Check sheet for the modelled part. Datum: model origin and axes. Units: mm. A direction names the side the tool comes from. Round coordinates to 2 decimals unless told otherwise and drop trailing zeros. Loops run counter-clockwise (first coordinate to the right, second up) from the corner with the lowest first, then second, coordinate; pieces in that order, holes last. Notation, with made-up numbers: (73, 5) - (87, 5) arc R16 cw to (87, 14) - close; hole circle Ø5 at (81.5, 48). An arc over 180 degrees is marked (long way). Put each result on its own line as item: value. Start each with the question number.
Item 1: Draft check along X on faces 4 (the conical face through (-34.97, -0.09, 75.19)), 5 (the conical face through (-37.42, -0.09, 77.21)), 6 (the flat face through (6.123, 34.723, 75.862)). Enter one of: pulls with the +X half, pulls with the -X half, needs draft (parallel to the pull), parting line crosses it, or undercut.
Item 2: Section check C-C, the plane x = -18.5. Record the cut outline in (y, z), and give its area (3 significant figures).
Item 3: Gauge pin test, flat ends, axial feed: pin 1 Ø23 at (x, y) = (-13, -16) entering from -Z; pin 2 Ø5 at (x, z) = (4.5, 47.5) entering from -Y; pin 3 Ø4 at (x, z) = (1.5, 152) entering from +Y (3 decimals); pin 4 Ø1.5 at (x, z) = (-31.5, 93.5) entering from +Y. Record the tip position at first contact, or that the pin passes through.
Item 4: Material ranges on line 1 along Y through (x, z) = (0, 154) (3 decimals); line 2 along Y through (x, z) = (0, -1.75) (3 decimals); line 3 along X through (y, z) = (0, 0), recorded low to high.
Item 5: Section check B-B, the plane y = 0. Record the cut outline in (x, z).
Item 6: Section check D-D, the plane y = -27. Record the cut outline in (x, z), and give its area (3 significant figures).
Item 7: Tool access check on faces 1 (the flat face through (-35.99, 6.346, 75.862)), 2 (the flat face through (0, 38.735, 0)), 3 (the conical face through (34.97, 0.09, 75.19)). Record the directions out of +Z, -Z, +X, -X, +Y, -Y that give a thin tool (end or side, any length) a straight path to the whole face; none if there is none.
Item 8: Section check A-A, the plane z = 110. Record the cut outline in (x, y).
from build123d import *

# Parameters (mm, degrees)
SKETCH1_R                      = 40.64
SKETCH1_R_2                    = 38.1
BOSS_EXTRUDE1_DEPTH            = 3.81
CUT_EXTRUDE1_REACH             = 5.81
SKETCH2_W                      = 7.62
SKETCH2_H                      = 3.81
CUT_EXTRUDE1_DIRECTION_2_REACH = 5.81
SKETCH3_R                      = 34.29
SKETCH3_R_2                    = 31.75
BOSS_EXTRUDE2_DEPTH            = 3.81
REVOLVE1_ANGLE                 = 10
REVOLVE1_OTHER_WAY_ANGLE       = 10
CUT_EXTRUDE2_REACH             = 162.02
SKETCH6_W                      = 7.62
SKETCH6_H                      = 3.81
REVOLVE2_ANGLE                 = 10
REVOLVE2_OTHER_WAY_ANGLE       = 10


with BuildPart() as part:
    # Sketch1 → Boss-Extrude1 (new body, symmetric)
    with BuildSketch(Plane.XY):
        Circle(SKETCH1_R)
        Circle(SKETCH1_R_2, mode=Mode.SUBTRACT)
    extrude(amount=BOSS_EXTRUDE1_DEPTH, both=True)

    # Sketch2 → Cut-Extrude1 (cut, up to next)
    with BuildSketch(Plane.XY, mode=Mode.PRIVATE) as cut_extrude1_sk1:
        with Locations((0, 40.64)):
            Rectangle(SKETCH2_W, SKETCH2_H)
    cut_extrude1_tool1 = extrude(cut_extrude1_sk1.sketch, amount=-CUT_EXTRUDE1_REACH, mode=Mode.PRIVATE) & part.part
    add(cut_extrude1_tool1.solids().sort_by_distance((0, 40.64, 0))[0], mode=Mode.SUBTRACT)

    # Sketch2 → Cut-Extrude1 direction 2 (cut, up to next)
    with BuildSketch(Plane.XY, mode=Mode.PRIVATE) as cut_extrude1_direction_2_sk1:
        with Locations((0, 40.64)):
            Rectangle(SKETCH2_W, SKETCH2_H)
    cut_extrude1_direction_2_tool1 = extrude(cut_extrude1_direction_2_sk1.sketch, amount=CUT_EXTRUDE1_DIRECTION_2_REACH, mode=Mode.PRIVATE) & part.part
    add(cut_extrude1_direction_2_tool1.solids().sort_by_distance((0, 40.64, 0))[0], mode=Mode.SUBTRACT)



with BuildPart() as body_2:
    # Sketch3 → Boss-Extrude2 (new body, symmetric)
    with BuildSketch(Plane.XY.offset(152.4)):
        Circle(SKETCH3_R)
        Circle(SKETCH3_R_2, mode=Mode.SUBTRACT)
    extrude(amount=BOSS_EXTRUDE2_DEPTH, both=True)


with BuildPart() as part_1:
    add(part.part)

    add(body_2.part)  # Revolve1 merges body 2
    # Sketch5 → Revolve1 (revolve)
    with BuildSketch(Plane(origin=(0, 0, 0), x_dir=(1, 0, 0), z_dir=(0, 1, 0))):
        Polygon((-40.64, -3.81), (-34.29, -148.59), (-31.75, -148.59), (-38.1, -3.81), align=None)
        Polygon((40.64, -3.81), (34.29, -148.59), (31.75, -148.59), (38.1, -3.81), align=None)
    revolve(axis=Axis((0, 0, -17.154345007), (0, 0, 1)), revolution_arc=REVOLVE1_ANGLE)

    # Sketch5 → Revolve1 other way (revolve)
    with BuildSketch(Plane(origin=(0, 0, 0), x_dir=(1, 0, 0), z_dir=(0, 1, 0))):
        Polygon((-40.64, -3.81), (-34.29, -148.59), (-31.75, -148.59), (-38.1, -3.81), align=None)
        Polygon((40.64, -3.81), (34.29, -148.59), (31.75, -148.59), (38.1, -3.81), align=None)
    revolve(axis=Axis((0, 0, -17.154345007), (0, 0, -1)), revolution_arc=REVOLVE1_OTHER_WAY_ANGLE)

    # Sketch6 → Cut-Extrude2 (cut, up to next)
    with BuildSketch(Plane.XY.offset(156.21), mode=Mode.PRIVATE) as cut_extrude2_sk1:
        with Locations((0, 34.29)):
            Rectangle(SKETCH6_W, SKETCH6_H)
    cut_extrude2_tool1 = extrude(cut_extrude2_sk1.sketch, amount=-CUT_EXTRUDE2_REACH, mode=Mode.PRIVATE) & part_1.part
    add(cut_extrude2_tool1.solids().sort_by_distance((0, 34.29, 156.21))[0], mode=Mode.SUBTRACT)

    # Sketch11 → Revolve2 (revolve)
    with BuildSketch(Plane(origin=(0, 0, 0), x_dir=(0, 0, -1), z_dir=(1, 0, 0))):
        Polygon((-148.59, 32.385), (-3.81, 38.735), (-3.81, 38.1), (-148.59, 31.75), align=None)
    revolve(axis=Axis((0, 0, 0), (0, 0, 1)), revolution_arc=REVOLVE2_ANGLE)

    # Sketch11 → Revolve2 other way (revolve)
    with BuildSketch(Plane(origin=(0, 0, 0), x_dir=(0, 0, -1), z_dir=(1, 0, 0))):
        Polygon((-148.59, 32.385), (-3.81, 38.735), (-3.81, 38.1), (-148.59, 31.75), align=None)
    revolve(axis=Axis((0, 0, 0), (0, 0, -1)), revolution_arc=REVOLVE2_OTHER_WAY_ANGLE)


solid = part_1.part
Check result:
1. face 4: undercut
1. face 5: pulls with the -X half
1. face 6: pulls with the +X half
2. outline: (-36.19, -3.81) - (-33.31, -3.81) - (-33.31, 3.81) - (-36.19, 3.81) - close; (-28.87, 148.59) - (-25.8, 148.59) - (-25.8, 156.21) - (-28.87, 156.21) - close; (25.8, 148.59) - (28.87, 148.59) - (28.87, 156.21) - (25.8, 156.21) - close; (33.31, -3.81) - (36.19, -3.81) - (36.19, 3.81) - (33.31, 3.81) - close
2. area: 90.6 mm²
3. pin 1: z = 148.59
3. pin 2: y = 35.56
3. pin 3: y = 32.385
3. pin 4: through
4. line 1: -34.29 to -31.75, 31.75 to 32.385
4. line 2: -40.64 to -38.1, 38.1 to 38.735
4. line 3: -40.64 to -38.1, 38.1 to 40.64
5. outline: (-40.64, -3.81) - (-38.1, -3.81) - (-38.1, 3.81) - (-31.75, 148.59) - (-31.75, 156.21) - (-34.29, 156.21) - (-34.29, 148.59) - (-40.64, 3.81) - close; (31.75, 148.59) - (38.1, 3.81) - (38.1, -3.81) - (40.64, -3.81) - (40.64, 3.81) - (34.29, 148.59) - (34.29, 156.21) - (31.75, 156.21) - close
6. outline: (-30.37, -3.81) - (-26.88, -3.81) - (-26.88, 3.81) - (-30.37, 3.81) - close; (-21.14, 148.59) - (-16.71, 148.59) - (-16.71, 156.21) - (-21.14, 156.21) - close; (16.71, 148.59) - (21.14, 148.59) - (21.14, 156.21) - (16.71, 156.21) - close; (26.88, -3.81) - (30.37, -3.81) - (30.37, 3.81) - (26.88, 3.81) - close
6. area: 121 mm²
7. face 1: +Y
7. face 2: +Z, -Z, +Y
7. face 3: -Z
8. outline: (-35.44, -6.25) - (-32.93, -5.81) arc R33.44 cw to (-32.93, 5.81) - (-35.44, 6.25) arc R35.98 ccw to start; (-5.92, 33.56) - (-5.81, 32.93) arc R33.44 cw to (5.81, 32.93) - (5.92, 33.56) arc R34.08 ccw to start; (32.93, -5.81) - (35.44, -6.25) arc R35.98 ccw to (35.44, 6.25) - (32.93, 5.81) arc R33.44 cw to start
